Autodesk Inventor part; units mm, degrees
ref_plane "YZ Plane" through (0, 0, 0) normal (1, 0, 0) x (0, 1, 0)
ref_plane "XZ Plane" through (0, 0, 0) normal (0, 1, 0) x (-1, 0, 0)
ref_plane "XY Plane" through (0, 0, 0) normal (0, 0, 1) x (1, 0, 0)
sketch "Szkic1" plane through (0, 0, 0) normal (0, 0, 1) x (1, 0, 0)
  line L0 (0, 0) -> (40, 0)
  line L1 (40, 0) -> (40, 30)
  line L2 (40, 30) -> (0, 30)
  line L3 (0, 30) -> (0, 0)
  dimension "d0" = 40
  dimension "d1" = 30
extrude "Wyciągnięcie proste1" add sketch "Szkic1" along normal blind 5
sketch "Szkic2" plane through (0, 0, 5) normal (0, 0, 1) x (1, 0, 0)
  line L0 (40, 30) -> (0, 30)
  line L1 (0, 30) -> (40, 30)
  line L2 (40, 30) -> (40, 25)
  line L3 (40, 25) -> (0, 25)
  line L4 (0, 30) -> (0, 0)
  dimension "d4" = 5
extrude "Wyciągnięcie proste2" add sketch "Szkic2" along normal blind 30
sketch "Szkic5" plane through (0, 0, 0) normal (0, 0, -1) x (-1, 0, 0)
  line L0 (-40, 0) -> (-40, 25)
  line L1 (-40, 0) -> (0, 0)
  line L2 (0, 0) -> (0, -5)
  line L3 (0, -5) -> (-40, -5)
  line L4 (-40, -5) -> (-40, 0)
  dimension "d7" = 5
extrude "Wyciągnięcie proste3" add sketch "Szkic5" against normal blind 20
sketch "Szkic6" plane through (0, 25, 5) normal (0, -1, 0) x (1, 0, 0)
  point P0 (0, -5)
  point P1 (20, 21.543)
hole "Otwór1" at (20, 25, 26.543) direction (0, 1, 0) diameter 4 end through all
sketch "Szkic7" plane through (0, 25, 5) normal (0, -1, 0) x (1, 0, 0)
  circle A0 centre (20, 21.543) radius 2
  circle A1 centre (20, 21.543) radius 3
  point P0 (0, -5)
  dimension "d17" = 6
extrude "Wyciągnięcie proste4" cut sketch "Szkic7" against normal blind 2 contours A0 | A1
sketch "Szkic8" plane through (0, 0, 0) normal (0, 0, -1) x (-1, 0, 0)
  line L0 (-40, -5) -> (-40, 30)
  line L1 (0, 30) -> (0, -5)
  point P0 (0, 0)
  point P1 (-37, -2.5)
  point P2 (-3, -2.5)
  dimension "d20" = 3
  dimension "d21" = 3
hole "Otwór2" at (37, -2.5, 0) at (3, -2.5, 0) direction (0, 0, 1) diameter 2.9 end through all
properties part number "zacisk"
The listing builds one solid part. Answer for the finished solid, in the listing's coordinates (mm). A direction names the side the tool comes from. Give positions to 0.01 mm unless a question says otherwise; leave off trailing zeros. Write each loop counter-clockwise with the first axis right and the second up, starting at its lowest first coordinate (ties: lowest second). Pieces come first, ordered by that corner, then holes.
Item 1: Which of the six approach directions +Z, -Z, +X, -X, +Y, -Y give full straight-line access (tool end or side, diameter ignored) to faces 1 (the flat face through (20, 0, 12)), 2 (the cylindrical face through (19.609, 25.986, 29.517)), 3 (the flat face through (20, -2, 20))?
Item 2: Section A-A, the plane x = 20 is taken. Write down the section's boundary in (y, z), plus the area to 3 significant figures.
Item 3: Section C-C, the plane y = -2.5 is taken. Write down the section's boundary in (x, z), plus the area to 3 significant figures.
Item 4: Determine the mould class of faces 4 (the flat face through (20, 25, 20)), 5 (the flat face through (20, 27, 29)), 6 (the flat face through (20, 13, 5)) for opening direction Z: released by +Z, released by -Z, zero draft, split by the parting line, or undercut.
Item 5: Section B-B, the plane z = 15.5 is taken. Write down the section's boundary in (x, y).
Item 6: Flat-ended cylindrical pins translate along their axes: P1, Ø9, axis at x = 17.5, z = 27, coming from the -Y side; P2, Ø4, axis at x = 32.5, y = 24.5, coming from the +Z side; P3, Ø3, axis at x = 19.5, z = 25.5, coming from the -Y side; P4, Ø4.5, axis at x = 3, y = -2.5, coming from the +Z side. Find the tip coordinate at first contact, or state that the pin passes through.
Item 7: Find the intervals of material crossed by line 1 along X through (y, z) = (-2.5, 7); line 2 along Y through (x, z) = (37, 9.5); line 3 along Y through (x, z) = (4, 8), in increasing order.
Item 8: Section D-D, the plane x = 5.5 is taken. Write down the section's boundary in (y, z), plus the area to 3 significant figures.
Completed:
1. face 1: +Z, +X, -X
1. face 2: -Y
1. face 3: +Z, +X, -X, -Y
2. outline: (-5, 0) - (30, 0) - (30, 24.54) - (27, 24.54) - (27, 23.54) - (25, 23.54) - (25, 5) - (0, 5) - (0, 20) - (-5, 20) - close; (25, 29.54) - (27, 29.54) - (27, 28.54) - (30, 28.54) - (30, 35) - (25, 35) - close
2. area: 376 mm2
3. outline: (0, 0) - (1.55, 0) - (1.55, 20) - (0, 20) - close; (4.45, 0) - (35.55, 0) - (35.55, 20) - (4.45, 20) - close; (38.45, 0) - (40, 0) - (40, 20) - (38.45, 20) - close
3. area: 684 mm2
4. face 4: zero draft
4. face 5: undercut
4. face 6: released by +Z
5. outline: (0, -5) - (40, -5) - (40, 0) - (0, 0) - close; (0, 25) - (40, 25) - (40, 30) - (0, 30) - close; hole circle Ø2.9 at (3, -2.5); hole circle Ø2.9 at (37, -2.5)
6. P1: stops at y = 25
6. P2: stops at z = 35
6. P3: stops at y = 27
6. P4: stops at z = 20
7. line 1: x = 0 to 1.55, 4.45 to 35.55, 38.45 to 40
7. line 2: y = -5 to -3.95, -1.05 to 0, 25 to 30
7. line 3: y = -5 to -3.55, -1.45 to 0, 25 to 30
8. outline: (-5, 0) - (30, 0) - (30, 35) - (25, 35) - (25, 5) - (0, 5) - (0, 20) - (-5, 20) - close
8. area: 400 mm2
